For this review, take the finished solid that the model builds, in its own axes (mm). A direction names the side the tool comes from. Round coordinates to 2 decimals unless told otherwise and drop trailing zeros. Loops run counter-clockwise (first coordinate to the right, second up) from the corner with the lowest first, then second, coordinate; pieces in that order, holes last.
1) Wall thickness on L1, parallel to Y at x = 1.65, z = -0.8; L2, parallel to X at y = -1.45, z = -0.1; L3, parallel to Z at x = 1.35, y = -3.1: over which ranges is each line inside the solid? List them lowest first.
2) Insertion check: pin 1 (0.5 mm diameter, centred on y = -4.5, z = -0.5, fed in from +X); pin 2 (1.5 mm diameter, centred on y = -2, z = 1.5, fed in from +X); pin 3 (1.5 mm diameter, centred on x = 1.5, y = -2.5, fed in from -Z). Each pin has a flat end and moves straight along its axis. Give the tip position at first contact, or say it passes through.
3) Take a section at B-B (y = -3.1). State the section outline as (x, z) points, then the cut area to 3 significant figures.
4) Tool access review of faces 1 (the flat face through (3, -4.4, -0.3)), 2 (the flat face through (2, -5, 1)): name each direction out of +Z, -Z, +X, -X, +Y, -Y from which nothing blocks a thin tool from reaching the whole face with its end or side.
5) Take a section at C-C (z = 0.1). State the section outline as (x, y) points.
6) Take a section at A-A (x = 1.95). State the section outline as (y, z) points (3 decimals), then the cut area to 3 significant figures.
7) Take a section at D-D (x = 0.6). State the section outline as (y, z) points (3 decimals).
```python
from build123d import *

# Parameters (mm, degrees)
F1_DEPTH = 5
F2_DEPTH = 1
F4_DEPTH = 25


with BuildPart() as f1:
    # F0 (on Front) → F1 (new body)
    with BuildSketch(Plane.XZ):
        Polygon((3.25, 3.7996710384), (0, 0), (3, 0), (4.25, 3.7996710384), align=None)
    extrude(amount=F1_DEPTH)

    # F2 (add): a face of the model
    f2_faces = [f1.faces().sort_by_distance(p)[0] for p in [
        (1.5, -2.5, 0),
    ]]
    extrude(f2_faces, amount=F2_DEPTH)

    # F3 (on face) → F4 (cut)
    with BuildSketch(Plane(origin=(0, 0, 0), x_dir=(0, -1, 0), z_dir=(-1, 0, 0))):
        with BuildLine():
            Line((0, -1), (5, -1))
            ThreePointArc((5, -1), (3.8462912018, -0.2592719955), (2.5, 0))
            ThreePointArc((2.5, 0), (1.1537087982, -0.2592719955), (0, -1))
        make_face()
    extrude(amount=-F4_DEPTH, mode=Mode.SUBTRACT)


solid = f1.part
```
Response:
1. L1: y = -5 to -4.77, -0.23 to 0
1. L2: x = 0 to 3
1. L3: z = -0.05 to 1.58
2. pin 1: stops at x = 3
2. pin 2: stops at x = 3.74
2. pin 3: stops at z = -0.08
3. outline: (0, -0.05) - (3, -0.05) - (3, 0) - (4.25, 3.8) - (3.25, 3.8) - (0, 0) - close
3. area: 7.75 mm2
4. face 1: -Z, +X, +Y, -Y
4. face 2: +Z, -Z, +X, -X, -Y
5. outline: (0.09, -5) - (3.03, -5) - (3.03, 0) - (0.09, 0) - close
6. outline: (-5, -1) arc R3.625 cw to (0, -1) - (0, 2.28) - (-5, 2.28) - close
6. area: 13.0 mm2
7. outline: (-5, -1) arc R3.625 cw to (0, -1) - (0, 0.701) - (-5, 0.701) - close
